Input: dimensioned drawing with shaded views. Units: mm. Origin: part minimum x, y, z. A direction names the side the tool comes from. Round coordinates to 2 decimals unless told otherwise and drop trailing zeros. Loops run counter-clockwise (first coordinate to the right, second up) from the corner with the lowest first, then second, coordinate; pieces in that order, holes last. Notation, with made-up numbers: (29.25, 2) - (36.25, 2) arc R21 ccw to (36.25, 27) - close; hole circle Ø8 at (9, 71). An arc over 180 degrees is marked (long way). One line per question, with ' | ' between items. Start each with the question number.
1. Access query for the marked faces 5 and 6. Directions: +Z, -Z, +X, -X, +Y, -Y. A direction counts if a zero-diameter tool reaches every point of the face in a straight line with its end or side. Return the directions, or none.
2. Cut plane D-D (z = 21.5). Return loops of the section in (x, y), then the cut area to 3 significant figures.
3. Cut plane A-A (z = 49). Return loops of the section in (x, y) (1 decimal).
4. Ray query, line 1 (X direction, y = 23, z = 48); line 2 (Y direction, x = 125, z = 53.5); line 3 (Y direction, x = 131, z = 31). Return the intervals inside material, ascending.
5. Mould query, pull axis Y, two halves, no side actions, for the marked faces 1, 2, 3 and 4. Classes: pulls with the +Y half, pulls with the -Y half, needs draft (parallel to the pull), parting line crosses it, or undercut.
6. Pin query (flat end, axial travel): pin 1 (2.5 mm diameter, centred on x = 56, y = 69, fed in from +Z). Return the tip coordinate at first contact, or that it passes through.
7. Cut plane B-B (x = 8). Return loops of the section in (y, z), then the cut area to 3 significant figures.
8. Cut plane C-C (y = 15). Return loops of the section in (x, z).
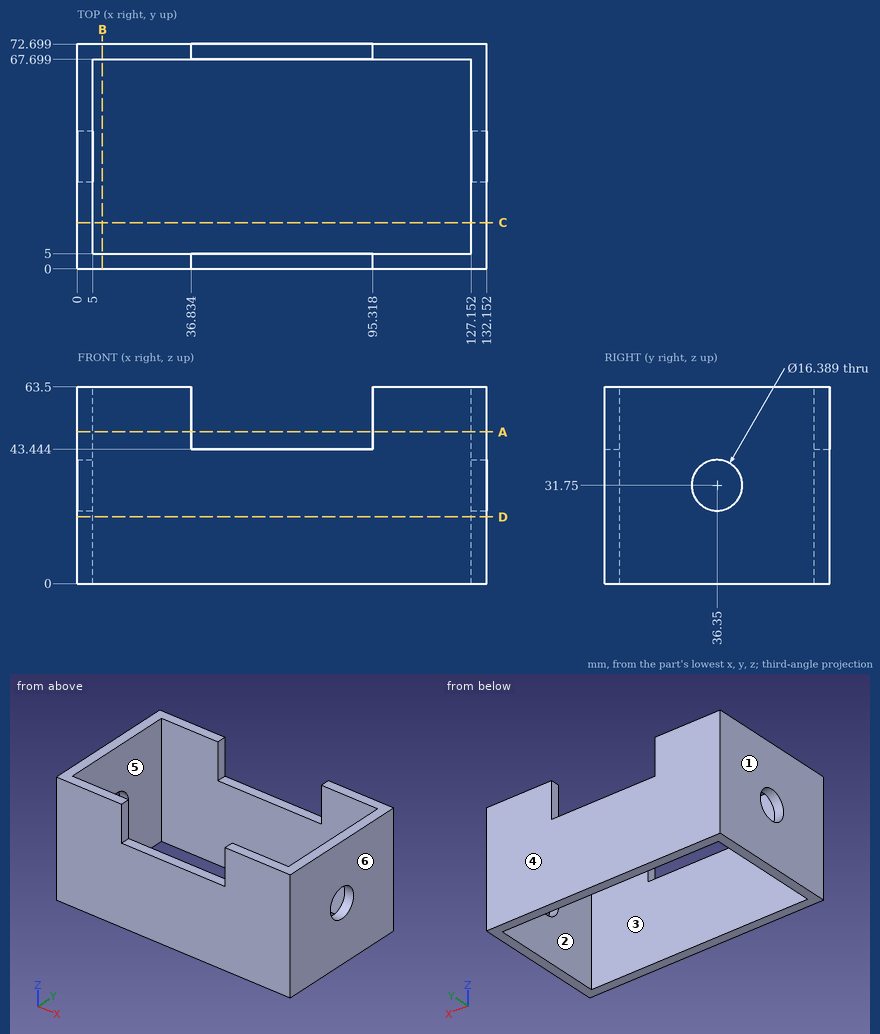
Answers follow:
1) face 5: +Z, -Z | face 6: +Z, -Z, +X, +Y, -Y
2) outline: (0, 0) - (132.15, 0) - (132.15, 72.7) - (0, 72.7) - close; hole (5, 5) - (127.15, 5) - (127.15, 67.7) - (5, 67.7) - close | area: 1,950 mm2
3) outline: (0, 0) - (36.8, 0) - (36.8, 5) - (5, 5) - (5, 67.7) - (36.8, 67.7) - (36.8, 72.7) - (0, 72.7) - close; (95.3, 0) - (132.2, 0) - (132.2, 72.7) - (95.3, 72.7) - (95.3, 67.7) - (127.2, 67.7) - (127.2, 5) - (95.3, 5) - close
4) line 1: x = 0 to 5, 127.15 to 132.15 | line 2: y = 0 to 5, 67.7 to 72.7 | line 3: y = 0 to 28.19, 44.51 to 72.7
5) face 1: needs draft | face 2: undercut | face 3: undercut | face 4: pulls with the +Y half
6) pin 1: stops at z = 43.44
7) outline: (0, 0) - (5, 0) - (5, 63.5) - (0, 63.5) - close; (67.7, 0) - (72.7, 0) - (72.7, 63.5) - (67.7, 63.5) - close | area: 635 mm2
8) outline: (0, 0) - (5, 0) - (5, 63.5) - (0, 63.5) - close; (127.15, 0) - (132.15, 0) - (132.15, 63.5) - (127.15, 63.5) - close
